Work out the finished part from the listing and answer in its coordinate system (mm). A direction names the side the tool comes from. Coordinates: 2 decimals unless noted, no trailing zeros. Write each loop counter-clockwise with the first axis right and the second up, starting at its lowest first coordinate (ties: lowest second). Pieces come first, ordered by that corner, then holes. Notation, with made-up numbers: M -12,16.25 L 2,16.25 A25 ccw 2,36.25 Z; hole C 4.25,55.25 d11. An arc over 180 degrees is marked long. Answer as CSV lines item,"result". Start each with the question number.
(1) Find the intervals of material crossed by L1, parallel to X at y = -6.25, z = 0; L2, parallel to Y at x = 27.5, z = 44; L3, parallel to Z at x = -5.5, y = -8.5, in increasing order. Write a range as [from, to].
(2) Flat-ended cylindrical pins translate along their axes: P1, Ø3, axis at x = -31.5, y = -11.5, coming from the -Z side; P2, Ø1.5, axis at x = 11, z = 27.5, coming from the -Y side; P3, Ø4, axis at x = -12.5, z = 0, coming from the -Y side; P4, Ø4.5, axis at x = -33.59, z = -33.59, coming from the -Y side. Find the tip coordinate at first contact, or state that the pin passes through.
(3) For faces 1 (the flat face through (-34, 2, -34)), 2 (the flat face through (32.316, -2.864, 25.28)), 3 (the flat face through (-32.316, -2.969, 25.28)), 4 (the flat face through (-30, 0, 20)), determine the directions among +Z, -Z, +X, -X, +Y, -Y from which every point of the face is accessible in a straight line to the end or side of a thin tool.
(4) A cutting plane is placed at A-A on y = -9.75. Give the vertices of the cut face in (x, z).
(5) The mould has two halves that part along X. Classify faces 5 (the flat face through (35.761, 6.479, -48.182)), 6 (the conical face through (-29.19, -5.784, -29.309)), 7 (the flat face through (34, 2, 34)): released by +X, released by -X, zero draft, split by the parting line, or undercut.
from build123d import *

# Parameters (mm, degrees)
BOSS_EXTRUDE1_DEPTH                                 = 8
SKETCH2_R                                           = 3.875
SKETCH2_R_2                                         = 2.05
CUT_EXTRUDE1_DEPTH                                  = 103.661522502
CIRPATTERN1_COUNT                                   = 4
SKETCH4_R                                           = 34.5
SKETCH4_R_2                                         = 30.5
BOSS_EXTRUDE2_DEPTH                                 = 12.5
SKETCH5_R                                           = 20
BOSS_EXTRUDE3_DEPTH                                 = 1
SKETCH6_R                                           = 17.5
BOSS_EXTRUDE4_DEPTH                                 = 18
SKETCH7_R                                           = 7.5
CUT_EXTRUDE2_DEPTH                                  = 106.85078272
SKETCH9_R                                           = 3.975
BOSS_EXTRUDE6_DEPTH                                 = 2
SKETCH10_R                                          = 4.975
BOSS_EXTRUDE7_DEPTH                                 = 3
CHAMFER2_START                                      = -3.006253442
CHAMFER2_DEPTH                                      = 0.006253442
CHAMFER2_START_2                                    = -7.5000001
CHAMFER2_2_DEPTH                                    = 4.493746658
CHAMFER2_3_ANGLE                                    = 16.582247
CIRPATTERN2_COUNT                                   = 4
CSK_FOR_M4_COUNTERSUNK_FLAT_HEAD_SCREW1_D           = 3.6
CSK_FOR_M4_COUNTERSUNK_FLAT_HEAD_SCREW1_CSINK_D     = 9.1
CSK_FOR_M4_COUNTERSUNK_FLAT_HEAD_SCREW1_CSINK_ANGLE = 90
BOSS_EXTRUDE8_DEPTH                                 = 12.5
FILLET1_R                                           = 5


with BuildPart() as part:
    # Sketch1 → Boss-Extrude1 (new body)
    with BuildSketch(Plane(origin=(0, 0, 0), x_dir=(1, 0, 0), z_dir=(0, 1, 0))):
        Polygon((0, 74.16407865), (-70.534230275, 22.917960675), (-43.59255168, -60), (43.59255168, -60), (70.534230275, 22.917960675), align=None)
    extrude(amount=BOSS_EXTRUDE1_DEPTH)

    # Sketch2 → Cut-Extrude1 (cut, through all)
    with BuildSketch(Plane(origin=(0, 8, 0), x_dir=(1, 0, 0), z_dir=(0, 1, 0))):
        with Locations(Location((-33.587572106, -33.587572106, 0), (0, 0, 270))):
            Circle(SKETCH2_R)
        with Locations(Location((-43.487067043, -23.68807717, 0), (0, 0, 270))):
            Circle(SKETCH2_R_2)
        with Locations(Location((-23.68807717, -43.487067043, 0), (0, 0, 270))):
            Circle(SKETCH2_R_2)
        with Locations(Location((0, -49.52, 0), (0, 0, 270))):
            Circle(SKETCH2_R_2)
    cut_extrude1 = extrude(amount=-CUT_EXTRUDE1_DEPTH, mode=Mode.SUBTRACT)

    # CirPattern1: Cut-Extrude1 ×4 about axis
    cirpattern1_axis = Axis((0, 0, 0), (0, 1, 0))
    for i in range(1, CIRPATTERN1_COUNT):
        add(cut_extrude1.rotate(cirpattern1_axis, i * 360 / CIRPATTERN1_COUNT), mode=Mode.SUBTRACT)

    # Sketch4 → Boss-Extrude2 (add)
    with BuildSketch(Plane.XZ):
        with Locations(Location((0, 0, 0), (0, 0, 90))):
            Circle(SKETCH4_R)
        with Locations(Location((0, 0, 0), (0, 0, 270))):
            Circle(SKETCH4_R_2, mode=Mode.SUBTRACT)
    extrude(amount=BOSS_EXTRUDE2_DEPTH)

    # Sketch5 → Boss-Extrude3 (add)
    with BuildSketch(Plane.XZ):
        with Locations(Location((0, 0, 0), (0, 0, 90))):
            Circle(SKETCH5_R)
    extrude(amount=BOSS_EXTRUDE3_DEPTH)

    # Sketch6 → Boss-Extrude4 (add)
    with BuildSketch(Plane.XZ.offset(1)):
        with Locations(Location((0, 0, 0), (0, 0, 270))):
            Circle(SKETCH6_R)
    extrude(amount=BOSS_EXTRUDE4_DEPTH)

    # Sketch7 → Cut-Extrude2 (cut, through all)
    with BuildSketch(Plane.XZ.offset(19)):
        with Locations(Location((0, 0, 0), (0, 0, 270))):
            Circle(SKETCH7_R)
    extrude(amount=-CUT_EXTRUDE2_DEPTH, mode=Mode.SUBTRACT)

    # Sketch9 → Boss-Extrude6 (add)
    with BuildSketch(Plane.XZ):
        with Locations((33.587572106, -33.587572106)):
            Circle(SKETCH9_R)
        with Locations((-33.587572106, -33.587572106)):
            Circle(SKETCH9_R)
        with Locations((-33.587572106, 33.587572106)):
            Circle(SKETCH9_R)
        with Locations((33.587572106, 33.587572106)):
            Circle(SKETCH9_R)
    extrude(amount=-BOSS_EXTRUDE6_DEPTH)

    # Sketch10 → Boss-Extrude7 (add)
    with BuildSketch(Plane.XZ):
        with BuildLine():
            Line((20.6223527, -27.658065173), (30.06971587, -37.105428343))
            ThreePointArc((30.06971587, -37.105428343), (30.06971587, -30.06971587), (37.105428343, -30.06971587))
            Line((37.105428343, -30.06971587), (27.658065173, -20.6223527))
            ThreePointArc((27.658065173, -20.6223527), (24.395183951, -24.395183951), (20.6223527, -27.658065173))
        make_face()
        with Locations((33.587572106, -33.587572106)):
            Circle(SKETCH10_R)
    boss_extrude7 = extrude(amount=BOSS_EXTRUDE7_DEPTH)

    # Chamfer2: read off the stored shape, not the designer's step
    # Chamfer2 outline → Chamfer2 (add)
    with BuildSketch(Plane(origin=(0, 0, 0), x_dir=(1, 0, 0), z_dir=(0, 1, 0)).offset(CHAMFER2_START)):
        with BuildLine():
            ThreePointArc((37.105428343, 30.06971587), (37.105428343, 37.105428343), (30.06971587, 37.105428343))
            Line((30.06971587, 37.105428343), (20.6223527, 27.658065173))
            ThreePointArc((20.6223527, 27.658065173), (24.395183951, 24.395183951), (27.658065173, 20.6223527))
            Line((27.658065173, 20.6223527), (37.105428343, 30.06971587))
        make_face()
    chamfer2 = extrude(amount=CHAMFER2_DEPTH)

    # Chamfer2 2 outline → Chamfer2 2 (add)
    with BuildSketch(Plane(origin=(0, 0, 0), x_dir=(1, 0, 0), z_dir=(0, 1, 0)).offset(CHAMFER2_START_2)):
        with BuildLine():
            ThreePointArc((37.105428343, 30.06971587), (37.105428343, 37.105428343), (30.06971587, 37.105428343))
            Line((30.06971587, 37.105428343), (20.6223527, 27.658065173))
            ThreePointArc((20.6223527, 27.658065173), (24.395183951, 24.395183951), (27.658065173, 20.6223527))
            Line((27.658065173, 20.6223527), (37.105428343, 30.06971587))
        make_face()
    chamfer2_2 = extrude(amount=CHAMFER2_2_DEPTH)

    # Chamfer2 3 outline → Chamfer2 3 (revolve, cut)
    with BuildSketch(Plane(origin=(0, 0, 0), x_dir=(0.801683048491221, 0, -0.597749353627273), z_dir=(0.597749353627273, 0, 0.801683048491221))):
        Polygon((52.475017897, -3.006245526), (34.5, -7.5), (52.475, -7.5000001), align=None)
    chamfer2_3 = revolve(axis=Axis((0, 0, 0), (0, 1, 0)), revolution_arc=CHAMFER2_3_ANGLE, mode=Mode.SUBTRACT)

    # CirPattern2: Boss-Extrude7, Chamfer2, Chamfer2 2, Chamfer2 3 ×4 about axis
    cirpattern2_axis = Axis((0, 0, 0), (0, 1, 0))
    add([boss_extrude7.rotate(cirpattern2_axis, i * 360 / CIRPATTERN2_COUNT) for i in range(1, CIRPATTERN2_COUNT)])
    add([chamfer2.rotate(cirpattern2_axis, i * 360 / CIRPATTERN2_COUNT) for i in range(1, CIRPATTERN2_COUNT)])
    add([chamfer2_2.rotate(cirpattern2_axis, i * 360 / CIRPATTERN2_COUNT) for i in range(1, CIRPATTERN2_COUNT)])
    add([chamfer2_3.rotate(cirpattern2_axis, i * 360 / CIRPATTERN2_COUNT) for i in range(1, CIRPATTERN2_COUNT)], mode=Mode.SUBTRACT)

    # CSK for M4 Countersunk Flat Head Screw1 (through all)
    with Locations(Plane(origin=(0, 8, -12.5), x_dir=(0, 0, 1), z_dir=(0, 1, 0))):
        with Locations((0, 0), (12.5, 12.5), (25, 0), (12.5, -12.5)):
            CounterSinkHole(CSK_FOR_M4_COUNTERSUNK_FLAT_HEAD_SCREW1_D / 2, CSK_FOR_M4_COUNTERSUNK_FLAT_HEAD_SCREW1_CSINK_D / 2, counter_sink_angle=CSK_FOR_M4_COUNTERSUNK_FLAT_HEAD_SCREW1_CSINK_ANGLE)

    # Sketch13 → Boss-Extrude8 (add)
    with BuildSketch(Plane.XZ):
        with BuildLine():
            Line((-11.79321147, -32.421754475), (-12.732901193, -35.928724264))
            ThreePointArc((-12.732901193, -35.928724264), (-10.611580849, -39.602958878), (-6.937346235, -37.481638534))
            Line((-6.937346235, -37.481638534), (-5.997656512, -33.974668745))
            ThreePointArc((-5.997656512, -33.974668745), (-8.929257056, -33.324441007), (-11.79321147, -32.421754475))
        make_face()
    extrude(amount=BOSS_EXTRUDE8_DEPTH)

    # Fillet1
    fillet1_edges = [part.edges().sort_by_distance(p)[0] for p in [
        (57.063390978, 0, 18.541019662),
        (0, 0, 60),
        (-57.063390978, 0, 18.541019662),
        (-35.267115138, 0, -48.541019662),
        (35.267115138, 0, -48.541019662),
    ]]
    fillet(fillet1_edges, radius=FILLET1_R)


solid = part.part
Here are the results:
1,L1,"x = [-34.5, -30.5], [-17.5, -14.3], [-10.7, -7.5], [7.5, 10.7], [14.3, 17.5], [30.5, 34.5]"
1,L2,"y = [0, 8]"
1,L3,"z = [-34.06, -30], [-16.61, -5.1], [5.1, 16.61], [30, 34.06]"
2,P1,"stops at z = -17.04"
2,P2,"stops at y = 0"
2,P3,"stops at y = -19"
2,P4,"stops at y = -4.81"
3,face 1,"+Y"
3,face 2,"+X, -Y"
3,face 3,"-X, -Y"
3,face 4,"-Y"
4,outline,"C 0,0 d35; M -12.73,-35.93 A3 ccw -6.94,-37.48 L -6,-33.97 A34.5 ccw long -11.79,-32.42 Z; hole C 0,0 d61; hole C -12.5,0 d3.6; hole C 0,0 d15; hole C 0,-12.5 d3.6; hole C 0,12.5 d3.6; hole C 12.5,0 d3.6"
5,face 5,"released by +X"
5,face 6,"released by -X"
5,face 7,"undercut"
